Here's the drawing with two shaded views (mm, measured from the low corner). I have some questions. Coordinates: 2 decimals unless noted, no trailing zeros. Loops run counter-clockwise (first coordinate to the right, second up) from the corner with the lowest first, then second, coordinate; pieces in that order, holes last. Notation, with made-up numbers: M -17.75,-21.75 L -1.75,-21.75 A19 ccw -1.75,-15.75 Z; hole C 43,88.25 d2. An arc over 180 degrees is marked long. Return JSON: item names as keys, results as strings. Group by question number.
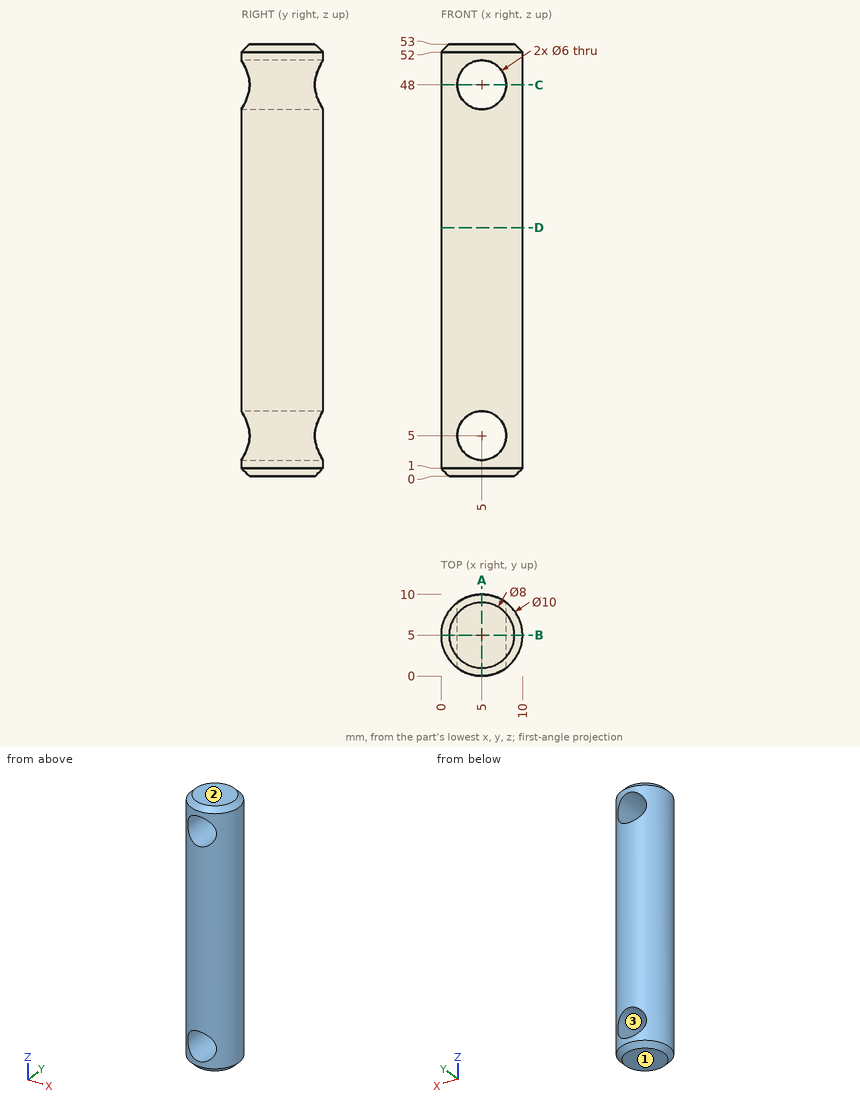
(1) Imagine slicing it at A-A, the plane x = 5. Write out the boundary of the cut face in (y, z), then the cut area to 3 significant figures.
(2) Will these pins go through, and if not, where does the flat tip stop? P1, Ø6, axis at x = 1.5, y = 7, coming from the -Z side; P2, Ø1.5, axis at x = 2, z = 17.5, coming from the -Y side; P3, Ø5.5, axis at x = 5, z = 5, coming from the +Y side; P4, Ø1, axis at x = 6.5, z = 31, coming from the -Y side.
(3) We'd pull the mould along Z, two halves only. Please class the marked faces 1, 2 and 3: +Z half, -Z half, draft (parallel to the pull), parting line (faces both ways), or undercut.
(4) Imagine slicing it at B-B, the plane y = 5. Write out the boundary of the cut face in (x, z), then the cut area to 3 significant figures.
(5) Imagine slicing it at C-C, the plane z = 48. Write out the boundary of the cut face in (x, y).
(6) If I drill on L1, parallel to Z at x = 3.75, y = 8.5; L2, parallel to Z at x = 7.5, y = 5.25; L3, parallel to Y at x = 1, z = 22, over which ranges is the centre line in solid material (lowest first)? Write a range as [from, to].
(7) Imagine slicing it at D-D, the plane z = 30.5. Write out the boundary of the cut face in (x, y).
Checks:
{
 "1": {"outline": "M 0,1 L 1,0 L 9,0 L 10,1 L 10,2 L 0,2 Z; M 0,8 L 10,8 L 10,45 L 0,45 Z; M 0,51 L 10,51 L 10,52 L 9,53 L 1,53 L 0,52 Z", "area": "408 mm²"},
 "2": {"P1": "z = 0", "P2": "y = 0.53", "P3": "through", "P4": "y = 0.1"},
 "3": {"face 1": "-Z half", "face 2": "+Z half", "face 3": "undercut"},
 "4": {"outline": "M 0,1 L 1,0 L 9,0 L 10,1 L 10,52 L 9,53 L 1,53 L 0,52 Z; hole C 5,5 d6; hole C 5,48 d6", "area": "471 mm²"},
 "5": {"outline": "M 2,1 L 2,9 A5 ccw Z; M 8,1 A5 ccw 8,9 Z"},
 "6": {"L1": "[0, 2.27], [7.73, 45.27], [50.73, 53]", "L2": "[0, 3.34], [6.66, 46.34], [49.66, 53]", "L3": "[2, 8]"},
 "7": {"outline": "C 5,5 d10"}
}
